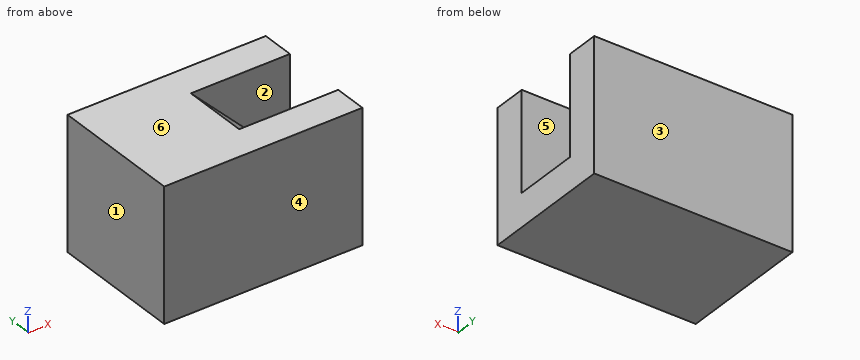
from build123d import *

# Parameters (mm, degrees)
F2_DEPTH = 25.4
F4_DEPTH = 25.4


with BuildPart() as f2:
    # F0 (on Front) → F2 (new body)
    with BuildSketch(Plane.XZ):
        Polygon((0, 25.4), (0, 0), (38.1, 0), (38.1, 6.35), (19.05, 25.4), align=None)
    extrude(amount=-F2_DEPTH)

    # F3 (on Top) → F4 (join)
    with BuildSketch(Plane.XY):
        Polygon((0, 25.4), (0, 0), (38.1, 0), (38.1, 6.35), (19.05, 6.35), (19.05, 19.05), (38.1, 19.05), (38.1, 25.4), align=None)
    extrude(amount=F4_DEPTH)


solid = f2.part
The listing builds one solid part. Answer for the finished solid, in the listing's coordinates (mm). Face numbers are marked on the shaded views. A direction names the side the tool comes from. Give positions to 0.01 mm unless a question says otherwise; leave off trailing zeros. Write each loop counter-clockwise with the first axis right and the second up, starting at its lowest first coordinate (ties: lowest second). Pieces come first, ordered by that corner, then holes. Notation, with made-up numbers: (-23, -9.5) -> (-15, -9.5) arc R20 ccw to (-15, -0.5) -> close; hole circle Ø8 at (-10.5, -29). An arc over 180 degrees is marked (long way). One line per question, with ' | ' between items. Start each with the question number.
1. For the marked faces 1 and 2, determine the directions among +Z, -Z, +X, -X, +Y, -Y from which every point of the face is accessible in a straight line to the end or side of a thin tool.
2. Section B-B (y = 14) is taken. Determine the outline of the cut face in (x, z), plus the area to 3 significant figures.
3. Section C-C (z = 14) is taken. Determine the outline of the cut face in (x, y).
4. Find the intervals of material crossed by probe 1 along Y at (x, z) = (28, 20.75); probe 2 along Z at (x, y) = (34.5, 14); probe 3 along Z at (x, y) = (20, 15.5), in increasing order.
5. For a pull along Y with two mould halves and no side action, classify the marked faces 3, 4, 5 and 6 as pulls with the +Y half, pulls with the -Y half, needs draft (parallel to the pull), parting line crosses it, or undercut.
6. Section A-A (x = 35.5) is taken. Determine the outline of the cut face in (y, z), plus the area to 3 significant figures.
Response values:
1) face 1: +Z, -Z, -X, +Y, -Y | face 2: +Z, +X
2) outline: (0, 0) -> (38.1, 0) -> (38.1, 6.35) -> (19.05, 25.4) -> (0, 25.4) -> close | area: 786 mm2
3) outline: (0, 0) -> (38.1, 0) -> (38.1, 6.35) -> (30.45, 6.35) -> (30.45, 19.05) -> (38.1, 19.05) -> (38.1, 25.4) -> (0, 25.4) -> close
4) probe 1: 0 to 6.35, 19.05 to 25.4 | probe 2: 0 to 9.95 | probe 3: 0 to 24.45
5) face 3: pulls with the +Y half | face 4: pulls with the -Y half | face 5: undercut | face 6: needs draft
6) outline: (0, 0) -> (25.4, 0) -> (25.4, 25.4) -> (19.05, 25.4) -> (19.05, 8.95) -> (6.35, 8.95) -> (6.35, 25.4) -> (0, 25.4) -> close | area: 436 mm2
